Design review of the part built by this model. Coordinates are the model's own, in mm. A direction names the side the tool comes from. Round coordinates to 2 decimals unless told otherwise and drop trailing zeros. Loops run counter-clockwise (first coordinate to the right, second up) from the corner with the lowest first, then second, coordinate; pieces in that order, holes last. Notation, with made-up numbers: M 20,-27 L 30,-27 A18 cw 30,-1 Z; hole C 22,21.5 d3. An arc over 180 degrees is marked long. Answer as CSV lines item,"result". Start each with the question number.
from build123d import *

# Parameters (mm, degrees)
SKETCH1_W               = 8
SKETCH1_H               = 8
BOSS_EXTRUDE1_DEPTH     = 3
CUT_EXTRUDE1_DEPTH      = 12.704699911
CUT_EXTRUDE1_DEPTH_BACK = 12.704699911
CUT_EXTRUDE2_DEPTH      = 11
SKETCH4_R               = 1.8
CUT_EXTRUDE3_DEPTH      = 0.8
SKETCH5_W               = 8
SKETCH5_H               = 1
BOSS_EXTRUDE2_DEPTH     = 2
FILLET1_R               = 4
SKETCH6_W               = 1.153846154
SKETCH6_H               = 1.153846154
CUT_EXTRUDE4_DEPTH      = 0.4


with BuildPart() as part:
    # Sketch1 → Boss-Extrude1 (new body)
    with BuildSketch(Plane(origin=(0, 0, 0), x_dir=(1, 0, 0), z_dir=(0, 1, 0))):
        with Locations((4, 4)):
            Rectangle(SKETCH1_W, SKETCH1_H)
    extrude(amount=BOSS_EXTRUDE1_DEPTH)

    # Sketch2 → Cut-Extrude1 (cut, two sides: drawn at the far end of the back side and taken through both)
    with BuildSketch(Plane.XY.offset(-CUT_EXTRUDE1_DEPTH_BACK)):
        Polygon((0, 0), (0.6, 3), (0, 3), align=None)
        Polygon((8, 0), (7.4, 3), (8, 3), align=None)
    extrude(amount=CUT_EXTRUDE1_DEPTH + CUT_EXTRUDE1_DEPTH_BACK, mode=Mode.SUBTRACT)

    # Sketch3 → Cut-Extrude2 (cut)
    with BuildSketch(Plane(origin=(0, 0, 0), x_dir=(0, 0, -1), z_dir=(1, 0, 0))):
        Polygon((0, 0), (0.6, 3), (0, 3), align=None)
        Polygon((8, 3), (7.4, 3), (8, 0), align=None)
    extrude(amount=CUT_EXTRUDE2_DEPTH, mode=Mode.SUBTRACT)

    # Sketch4 → Cut-Extrude3 (cut)
    with BuildSketch(Plane.XZ):
        with Locations(Location((4, -3.75, 0), (0, 0, 270))):
            Circle(SKETCH4_R)
    extrude(amount=-CUT_EXTRUDE3_DEPTH, mode=Mode.SUBTRACT)

    # Sketch5 → Boss-Extrude2 (add)
    with BuildSketch(Plane.XZ):
        with Locations((4, -7.5)):
            Rectangle(SKETCH5_W, SKETCH5_H)
    extrude(amount=BOSS_EXTRUDE2_DEPTH)

    # Fillet1
    # the kernel refuses this fillet: 4 mm, written as the material it takes off along each edge
    with BuildSketch(Plane(origin=(8, -2, -16.660254038), x_dir=(0, 1, 0), z_dir=(0, 0, 1)), Plane(origin=(0, -2, 1.660254038), x_dir=(0, 1, 0), z_dir=(0, 0, -1))) as fillet1_piece_1:
        with BuildLine():
            CenterArc((4, 3.464101615), FILLET1_R, 180, 60)
            Line((0, 3.464101615), (-0.08, 3.464101615))
            Line((-0.08, 3.464101615), (-0.08, 0))
            Line((-0.08, 0), (0, -0.08))
            ThreePointArc((0, -0.08), (1, -0.08), (1.96, -0.069282032))
            Line((1.96, -0.069282032), (2, 0))
        make_face()
    extrude(amount=18.320508076, mode=Mode.SUBTRACT)

    # Sketch6 → Cut-Extrude4 (cut)
    with BuildSketch(Plane(origin=(0, 3, 0), x_dir=(1, 0, 0), z_dir=(0, 1, 0))):
        with Locations((4.058809338, 4.067977948)):
            Rectangle(SKETCH6_W, SKETCH6_H)
    extrude(amount=-CUT_EXTRUDE4_DEPTH, mode=Mode.SUBTRACT)


solid = part.part
Item 1: Insertion check: pin 1 Ø2 at (x, y) = (6, 2) entering from +Z; pin 2 Ø2 at (x, z) = (4.5, -4.5) entering from -Y; pin 3 Ø1 at (x, z) = (5, -3) entering from -Y. Each pin has a flat end and moves straight along its axis. Give the tip position at first contact, or say it passes through.
Item 2: Consider section A-A, the plane y = 0.6. Write out the cut boundary in (x, z), then the cut area to 3 significant figures.
Item 3: To check wall thickness, follow line 1 (Y direction, x = 4.75, z = -5.5); line 2 (Z direction, x = 3.5, y = -1.2); line 3 (X direction, y = 0.25, z = -3.75). State the ranges of each line that lie inside material, in increasing order.
Item 4: Consider section D-D, the plane y = 1.5. Write out the cut boundary in (x, z).
Item 5: Consider section B-B, the plane x = 4. Write out the cut boundary in (y, z), then the cut area to 3 significant figures.
Item 6: The part is to be moulded in two halves that separate along Z. For faces 6 (the face through (3.9, 1.5, -7.7)), 7 (the face through (4.541, 0.394, -5.467)), 8 (the face through (3.9, 1.5, -0.3)), say which applies: +Z half, -Z half, draft (parallel to the pull), parting line (faces both ways), or undercut.
Item 7: Tool access review of faces 1 (the face through (4, -1, -7)), 2 (the face through (6.51, -1.48, -7.51)), 3 (the face through (4, 0.8, -4)), 4 (the face through (4, 2.6, -4)), 5 (the face through (7.7, 1.5, -4.1)): name each direction out of +Z, -Z, +X, -X, +Y, -Y from which nothing blocks a thin tool from reaching the whole face with its end or side.
Item 8: Consider section C-C, the plane z = -7.25. Write out the cut boundary in (x, y).
Found:
1,pin 1,"stops at z = -0.2"
1,pin 2,"stops at y = 0"
1,pin 3,"stops at y = 0.8"
2,outline,"M 0.12,-7.88 L 7.88,-7.88 L 7.88,-0.12 L 0.12,-0.12 Z; hole C 4,-3.75 d3.6"
2,area,"50.0 mm^2"
3,line 1,"y = 0 to 3"
3,line 2,"z = -8 to -7"
3,line 3,"x = 0.05 to 2.2, 5.8 to 7.95"
4,outline,"M 0.3,-7.7 L 7.7,-7.7 L 7.7,-0.3 L 0.3,-0.3 Z"
5,outline,"M -2,-8 L 0,-8 L 3,-7.4 L 3,-4.64 L 2.6,-4.64 L 2.6,-3.49 L 3,-3.49 L 3,-0.6 L 0,0 L 0,-1.95 L 0.8,-1.95 L 0.8,-5.55 L 0,-5.55 L 0,-7 L -2,-7 Z"
5,area,"20.9 mm^2"
6,face 6,"-Z half"
6,face 7,"undercut"
6,face 8,"+Z half"
7,face 1,"+Z, +X, -X, -Y"
7,face 2,"+Z, -Z, +X, -Y"
7,face 3,"-Y"
7,face 4,"+Y"
7,face 5,"+Z, -Z, +X, +Y"
8,outline,"M 0,0 A4 ccw 3.46,-2 L 4.54,-2 A4 ccw 8,0 L 7.4,3 L 0.6,3 Z"
